The listing builds one solid part. Answer for the finished solid, in the listing's coordinates (mm). Give positions to 0.01 mm unless a question says otherwise; leave off trailing zeros. Order: outer loops, then holes, each group sorted by start corner. A loop starts at its lowest first (then second) coordinate and runs counter-clockwise, first axis right, second up. Notation, with made-up numbers: (51, 25.5) - (95, 25.5) arc R18 cw to (95, 56.5) - close; hole circle Ø4 at (28, 56). An arc over 180 degrees is marked (long way). Answer as a JSON object with one key per item and string values. Group by question number.
Q1. A cutting plane is placed at C-C, the plane z = 5. Give the vertices of the cut face in (x, y), and give its area (3 significant figures).
Q2. A cutting plane is placed at D-D, the plane y = -8. Give the vertices of the cut face in (x, z), and give its area (3 significant figures).
Q3. Consider line 1 (X direction, y = 1.75, z = 0); line 2 (X direction, y = -5, z = -1). Determine where each line is inside the solid, lowest interval first.
Q4. The mould has two halves that part along X. Classify faces 1 (the face through (0, -10.315, 0)), 2 (the face through (-3.5, 0.1, -0.6)), 3 (the face through (-0.3, 0.1, -3.4)), 4 (the face through (-7.493, 0.144, -0.33)): released by +X, released by -X, zero draft, split by the parting line, or undercut.
Q5. Given pin 1 (1.7 mm diameter, centred on x = 0, z = 4.76, fed in from +Y); pin 2 (5 mm diameter, centred on y = -6, z = 3, fed in from +X); pin 3 (4 mm diameter, centred on x = -3.5, y = 2, fed in from -Z); pin 4 (1 mm diameter, centred on x = -5.5, y = -2, fed in from +Z), each flat-ended and moving along its own axis, determine where each tip first touches the part or whether it passes through.
Q6. A cutting plane is placed at A-A, the plane z = 0. Give the vertices of the cut face in (x, y), and give its area (3 significant figures).
Q7. A cutting plane is placed at B-B, the plane x = 0. Give the vertices of the cut face in (y, z).
from build123d import *

# Parameters (mm, degrees)
SKETCH2_R           = 7.5
BOSS_EXTRUDE1_DEPTH = 10.31494
SKETCH3_R           = 1.397
CUT_EXTRUDE1_DEPTH  = 11.31494
CIRPATTERN1_COUNT   = 4


with BuildPart() as part:
    # Sketch2 → Boss-Extrude1 (new body, symmetric)
    with BuildSketch(Plane(origin=(0, 0, 0), x_dir=(1, 0, 0), z_dir=(0, 1, 0))):
        Circle(SKETCH2_R)
    extrude(amount=BOSS_EXTRUDE1_DEPTH, both=True)

    # Sketch3 → Cut-Extrude1 (cut, symmetric)
    with BuildSketch(Plane(origin=(0, 0, 0), x_dir=(1, 0, 0), z_dir=(0, 1, 0))):
        with Locations((0, 4.7625)):
            Circle(SKETCH3_R)
    cut_extrude1 = extrude(amount=CUT_EXTRUDE1_DEPTH, both=True, mode=Mode.SUBTRACT)

    # CirPattern1: Cut-Extrude1 ×4 about axis
    cirpattern1_axis = Axis((0, 0, 0), (0, 1, 0))
    for i in range(1, CIRPATTERN1_COUNT):
        add(cut_extrude1.rotate(cirpattern1_axis, i * 360 / CIRPATTERN1_COUNT), mode=Mode.SUBTRACT)


solid = part.part
Reply:
{
 "1": {"outline": "(-5.59, -10.31) - (-1.38, -10.31) - (-1.38, 10.31) - (-5.59, 10.31) - close; (1.38, -10.31) - (5.59, -10.31) - (5.59, 10.31) - (1.38, 10.31) - close", "area": "174 mm^2"},
 "2": {"outline": "circle Ø15 at (0, 0); hole circle Ø2.79 at (-4.76, 0); hole circle Ø2.79 at (0, -4.76); hole circle Ø2.79 at (0, 4.76); hole circle Ø2.79 at (4.76, 0)", "area": "152 mm^2"},
 "3": {"line 1": "x = -7.5 to -6.16, -3.37 to 3.37, 6.16 to 7.5", "line 2": "x = -7.43 to -5.74, -3.79 to 3.79, 5.74 to 7.43"},
 "4": {"face 1": "zero draft", "face 2": "undercut", "face 3": "undercut", "face 4": "split by the parting line"},
 "5": {"pin 1": "passes through", "pin 2": "stops at x = 7.48", "pin 3": "stops at z = -7.35", "pin 4": "stops at z = 5.59"},
 "6": {"outline": "(-7.5, -10.31) - (-6.16, -10.31) - (-6.16, 10.31) - (-7.5, 10.31) - close; (-3.37, -10.31) - (3.37, -10.31) - (3.37, 10.31) - (-3.37, 10.31) - close; (6.16, -10.31) - (7.5, -10.31) - (7.5, 10.31) - (6.16, 10.31) - close", "area": "194 mm^2"},
 "7": {"outline": "(-10.31, -7.5) - (10.31, -7.5) - (10.31, -6.16) - (-10.31, -6.16) - close; (-10.31, -3.37) - (10.31, -3.37) - (10.31, 3.37) - (-10.31, 3.37) - close; (-10.31, 6.16) - (10.31, 6.16) - (10.31, 7.5) - (-10.31, 7.5) - close"}
}
